```python
from build123d import *

# Parameters (mm, degrees)
SKETCH_1_R          = 1.5
SKETCH_1_R_2        = 2
EXTRUDE_1_DEPTH     = 3
EXTRUDE_2_DEPTH     = 3
CUT_EXTRUDE_1_DEPTH = 112.846375834


with BuildPart() as part:
    # 草图1 → 凸台-拉伸1 (new body)
    with BuildSketch(Plane.XY):
        with BuildLine():
            Line((-46.419972715, 26.434696638), (-100.702636481, 42))
            Line((-100.702636481, 42), (-100.702636481, 48))
            Line((-100.702636481, 48), (100.702636481, 48))
            Line((100.702636481, 48), (100.702636481, 42))
            Line((100.702636481, 42), (46.419972715, 26.434696638))
            ThreePointArc((46.419972715, 26.434696638), (35.478614393, 20.327525063), (28.382623085, 10))
            Line((28.382623085, 10), (-28.382623085, 10))
            ThreePointArc((-28.382623085, 10), (-35.478614393, 20.327525063), (-46.419972715, 26.434696638))
        make_face()
        with Locations((-54, 37)):
            Circle(SKETCH_1_R, mode=Mode.SUBTRACT)
        with Locations((-35.5, 32.04293994)):
            Circle(SKETCH_1_R, mode=Mode.SUBTRACT)
        with Locations((-21.95706006, 18.5)):
            Circle(SKETCH_1_R, mode=Mode.SUBTRACT)
        with Locations(Location((21.95706006, 18.5, 0), (0, 0, 180))):
            Circle(SKETCH_1_R, mode=Mode.SUBTRACT)
        with Locations(Location((35.5, 32.04293994, 0), (0, 0, 180))):
            Circle(SKETCH_1_R, mode=Mode.SUBTRACT)
        with Locations(Location((54, 37, 0), (0, 0, 180))):
            Circle(SKETCH_1_R, mode=Mode.SUBTRACT)
        with Locations((-90, 44)):
            Circle(SKETCH_1_R_2, mode=Mode.SUBTRACT)
        with Locations((-70, 44)):
            Circle(SKETCH_1_R_2, mode=Mode.SUBTRACT)
        with Locations(Location((70, 44, 0), (0, 0, 180))):
            Circle(SKETCH_1_R_2, mode=Mode.SUBTRACT)
        with Locations(Location((90, 44, 0), (0, 0, 180))):
            Circle(SKETCH_1_R_2, mode=Mode.SUBTRACT)
    extrude(amount=EXTRUDE_1_DEPTH)

    # 草图2 → 凸台-拉伸2 (add)
    with BuildSketch(Plane.XY.offset(3)):
        Polygon((-100.702636481, 42), (-100.978273837, 41.038738304), (-67.334114479, 31.39143085), (-67.058477124, 32.352692546), align=None)
        Polygon((67.058477124, 32.352692546), (100.702636481, 42), (100.978273837, 41.038738304), (67.334114479, 31.39143085), align=None)
    extrude(amount=-EXTRUDE_2_DEPTH)

    # 草图3 → 切除-拉伸1 (cut, through all)
    with BuildSketch(Plane.XY.offset(3)):
        with BuildLine():
            Line((-6.641746516, 40.210125207), (-15.476556882, 19.658485028))
            ThreePointArc((-15.476556882, 19.658485028), (-17.211519663, 18.450985714), (-19.06092662, 19.474628401))
            ThreePointArc((-19.06092662, 19.474628401), (-30.09691848, 32.072460053), (-45.323396591, 39.047619048))
            ThreePointArc((-45.323396591, 39.047619048), (-46.877626016, 41.21821789), (-44.889566421, 43))
            Line((-44.889566421, 43), (-8.479162585, 43))
            ThreePointArc((-8.479162585, 43), (-6.808870756, 42.100056911), (-6.641746516, 40.210125207))
        make_face()
        with BuildLine():
            Line((-10.837416069, 17.789874793), (-1.837416069, 38.725781047))
            ThreePointArc((-1.837416069, 38.725781047), (0, 39.935906254), (1.837416069, 38.725781047))
            Line((1.837416069, 38.725781047), (10.837416069, 17.789874793))
            ThreePointArc((10.837416069, 17.789874793), (10.670291829, 15.899943089), (9, 15))
            Line((9, 15), (-9, 15))
            ThreePointArc((-9, 15), (-10.670291829, 15.899943089), (-10.837416069, 17.789874793))
        make_face()
        with BuildLine():
            Line((44.889566421, 43), (8.479162585, 43))
            ThreePointArc((8.479162585, 43), (6.808870756, 42.100056911), (6.641746516, 40.210125207))
            Line((6.641746516, 40.210125207), (15.476556882, 19.658485028))
            ThreePointArc((15.476556882, 19.658485028), (17.211519663, 18.450985714), (19.06092662, 19.474628401))
            ThreePointArc((19.06092662, 19.474628401), (30.09691848, 32.072460053), (45.323396591, 39.047619048))
            ThreePointArc((45.323396591, 39.047619048), (46.877626016, 41.21821789), (44.889566421, 43))
        make_face()
    extrude(amount=-CUT_EXTRUDE_1_DEPTH, mode=Mode.SUBTRACT)


solid = part.part
```
Geometry check sheet. Reference: the model listing, model coordinates, mm. A direction names the side the tool comes from. Give positions to 0.01 mm unless a question says otherwise; leave off trailing zeros. Order: outer loops, then holes, each group sorted by start corner. A loop starts at its lowest first (then second) coordinate and runs counter-clockwise, first axis right, second up. Notation, with made-up numbers: (67, -33.5) - (118, -33.5) arc R22 cw to (118, -13.5) - close; hole circle Ø4 at (2, 78.25). An arc over 180 degrees is marked (long way). Answer in a Markdown table with one row per item. Add a question column.
Q1. Cross-section at A-A, the plane x = 90. Enter the section's corners in (y, z), then the cut area to 3 significant figures.
Q2. Gauge pin test, flat ends, axial feed: pin 1 (2.5 mm diameter, centred on x = 70, y = 44, fed in from -Z); pin 2 (6.5 mm diameter, centred on x = -70, y = 44, fed in from -Z); pin 3 (0.9 mm diameter, centred on y = 43.5, z = 1, fed in from -X). Record the tip position at first contact, or that the pin passes through.
Q3. Cross-section at B-B, the plane z = 2.45. Count the separate pieces of the cut face and the enclosed holes in it, then the cut area to 3 significant figures.
Q4. Material ranges on probe 1 along Y at (x, z) = (-35.5, 0.9); probe 2 along X at (y, z) = (23, 2.8); probe 3 along Y at (x, z) = (-22, 0.4), recorded low to high. Write a range as from..to.
Q5. Mould release check, pull along Y, two halves, no side actions. Record for faces 1 (the flat face through (6.274, 28.404, 1.521)), 2 (the flat face through (-6.4, 28.11, 1.52)), 3 (the cylindrical face through (-35.35, 20.21, 1.48)), 4 (the flat face through (-1, 42, 3)): pulls with the +Y half, pulls with the -Y half, needs draft (parallel to the pull), parting line crosses it, or undercut.
Q6. Tool access check on faces 5 (the cylindrical face through (35.61, 20.446, 1.479)), 6 (the cylindrical face through (30, 32, 2)). Record the directions out of +Z, -Z, +X, -X, +Y, -Y that give a thin tool (end or side, any length) a straight path to the whole face; none if there is none.
Check values:
| question | item | result |
|---|---|---|
| 1 | outline | (37.89, 0) - (42, 0) - (42, 3) - (37.89, 3) - close; (46, 0) - (48, 0) - (48, 3) - (46, 3) - close |
| 1 | area | 18.3 mm^2 |
| 2 | pin 1 | passes through |
| 2 | pin 2 | stops at z = 0 |
| 2 | pin 3 | stops at x = -100.7 |
| 3 | separate pieces | 1 |
| 3 | enclosed holes | 13 |
| 3 | area | 3,300 mm^2 |
| 4 | probe 1 | y = 20.35..30.54, 33.54..35.46, 43..48 |
| 4 | probe 2 | x = -38.93..-21.27, -14.04..-8.6, 8.6..14.04, 21.27..38.93 |
| 4 | probe 3 | y = 10..17, 20..24, 43..48 |
| 5 | face 1 | undercut |
| 5 | face 2 | undercut |
| 5 | face 3 | pulls with the -Y half |
| 5 | face 4 | needs draft |
| 6 | face 5 | +Z, -Z, +X, -Y |
| 6 | face 6 | +Z, -Z |
